Geometry check sheet. Reference: drawing and pictorial views, mm from the part's lowest x, y, z. Coordinates: 2 decimals unless noted, no trailing zeros. Write each loop counter-clockwise with the first axis right and the second up, starting at its lowest first coordinate (ties: lowest second). Pieces come first, ordered by that corner, then holes. Notation, with made-up numbers: M 78,-15.5 L 133,-15.5 A13 cw 133,-10.5 Z; hole C 71.5,-37.5 d2. An arc over 180 degrees is marked long. One line per item, written item: value.
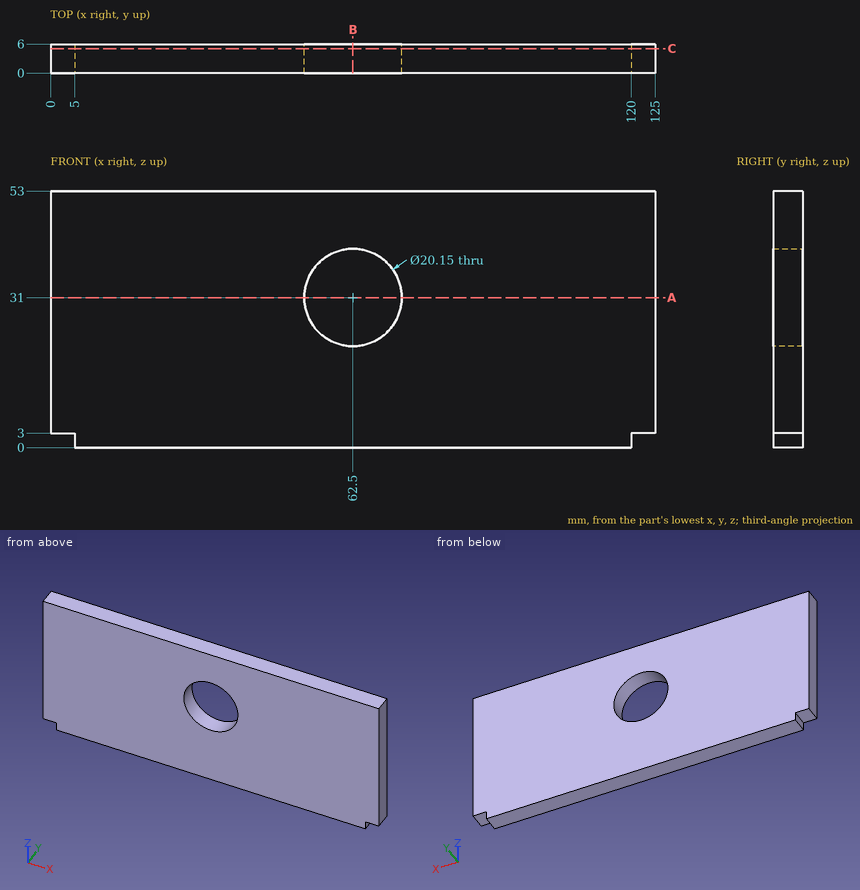
Item 1: Cross-section at B-B, the plane x = 62.5. Enter the section's corners in (y, z) (3 decimals), and give its area (3 significant figures).
The answers:
outline: M 0,0 L 6,0 L 6,20.925 L 0,20.925 Z; M 0,41.075 L 6,41.075 L 6,53 L 0,53 Z
area: 197 mm²
Item 2: Cross-section at C-C, the plane y = 5.05. Enter the section's corners in (x, z) (3 decimals), and give its area (3 significant figures).
The answers:
outline: M 0,3 L 5,3 L 5,0 L 120,0 L 120,3 L 125,3 L 125,53 L 0,53 Z; hole C 62.5,31 d20.15
area: 6,280 mm²
Item 3: Go/stop test with flat-tipped pins: P1, Ø1.5, axis at x = 123, y = 2, coming from the -Z side; P2, Ø2.5, axis at y = 2.5, z = 1.5, coming from the +X side; P3, Ø3.5, axis at y = 3, z = 1, coming from the -X side. Record where each tip stops, or that it passes through.
The answers:
P1: stops at z = 3
P2: stops at x = 120
P3: stops at x = 5
Item 4: Scan lines: line 1 (X direction, y = 3.15, z = 31) (3 decimals); line 2 (Z direction, x = 62.5, y = 1.2) (3 decimals); line 3 (X direction, y = 0.6, z = 33.5). Record each from-to range of solid material in increasing order.
The answers:
line 1: x = 0 to 52.425, 72.575 to 125
line 2: z = 0 to 20.925, 41.075 to 53
line 3: x = 0 to 52.74, 72.26 to 125
Item 5: Cross-section at A-A, the plane z = 31. Enter the section's corners in (x, y) (3 decimals).
The answers:
outline: M 0,0 L 52.425,0 L 52.425,6 L 0,6 Z; M 72.575,0 L 125,0 L 125,6 L 72.575,6 Z
